from build123d import *

# Parameters (mm, degrees)
F1_DEPTH = 20
F2_W     = 20
F2_H     = 20
F3_DEPTH = 20
F5_D     = 13.2
F7_DEPTH = 20


with BuildPart() as f1:
    # F0 (on Front) → F1 (new body)
    with BuildSketch(Plane.XZ):
        Polygon((-4.964183461, 2), (-4.964183461, 0), (2.535816539, 0), (2.535816539, 2), (6.453912527, 2), (6.453912527, 4), (2.535816539, 8), (-4.964183461, 8), (-8.8822794489, 4), (-8.8822794489, 2), align=None)
        Polygon((2.535816539, 0), (-4.964183461, 0), (-8.8822794489, 0), (-8.8822794489, -55), (6.453912527, -55), (6.453912527, 0), align=None)
    extrude(amount=F1_DEPTH)

    # F2 (on face) → F3 (join)
    with BuildSketch(Plane.YZ.offset(6.453912527)):
        with Locations((-10, -45)):
            Rectangle(F2_W, F2_H)
    extrude(amount=F3_DEPTH)

    # F5 (through all)
    with Locations(Plane.YZ.offset(26.453912527)):
        with Locations((-10, -45)):
            Hole(F5_D / 2)

    # F6 (on face) → F7 (join)
    with BuildSketch(Plane.XZ.offset(20)):
        Polygon((6.453912527, -35), (26.453912527, -35), (6.453912527, 0), align=None)
    extrude(amount=-F7_DEPTH)


solid = f1.part
Could you check a few things on this model? Use its own coordinates, in mm. A direction names the side the tool comes from. Give positions to 0.01 mm unless a question says otherwise; leave off trailing zeros. Order: outer loops, then holes, each group sorted by start corner. A loop starts at its lowest first (then second) coordinate and runs counter-clockwise, first axis right, second up.
Item 1: If we section it at B-B, the plane x = 5: Write out the boundary of the cut face in (y, z).
Item 2: For faces 1 (the face through (9, -10, -55)), 2 (the face through (-4.964, -10, 1)), 3 (the face through (6.454, -10, 3)), 4 (the face through (4, -10, 2)), 5 (the face through (-8.882, -10, 3)), which set-ups out of +Z, -Z, +X, -X, +Y, -Y let a thin tool reach every point of the face, with its end or its side?
Item 3: If we section it at C-C, the plane z = -45: Write out the boundary of the cut face in (x, y), plus the area to 3 significant figures.
Item 4: I'm going to push flat-ended pins straight in: pin 1 (8 mm diameter, centred on y = -10, z = -45, fed in from +X); pin 2 (1 mm diameter, centred on y = -10.5, z = 1, fed in from -X); pin 3 (2 mm diameter, centred on x = -6.5, y = -9, fed in from +Z); pin 4 (2 mm diameter, centred on x = 4.5, y = -12, fed in from +Z). Where does each tip first touch, or does it pass through?
Item 5: I need wall thicknesses on line 1 (Z direction, x = -1, y = -10); line 2 (Z direction, x = 3.5, y = -12.5); line 3 (Z direction, x = 5, y = -10). Which ranges of each line are inside material? Lowest first, please.
Item 6: If we section it at A-A, the plane y = -10: Write out the boundary of the cut face in (x, z).
Item 7: If we mould it in two halves opening along Z, with no side actions, what happens to faces 6 (the face through (5, -10, 0)), 7 (the face through (-6.896, -9.86, 6.028)), 8 (the face through (26.454, -17, -45)), 9 (the face through (8.538, -4.762, -49.016))? For each: pulls with the +Z half, pulls with the -Z half, needs draft (parallel to the pull), parting line crosses it, or undercut.
Item 8: If we section it at D-D, the plane x = 24: Write out the boundary of the cut face in (y, z), plus the area to 3 significant figures.
Values:
1. outline: (-20, -55) - (0, -55) - (0, 0) - (-20, 0) - close; (-20, 2) - (0, 2) - (0, 5.48) - (-20, 5.48) - close; hole circle Ø13.2 at (-10, -45)
2. face 1: -Z, +X, -X, +Y, -Y
2. face 2: -X, +Y, -Y
2. face 3: +Z, +X, +Y, -Y
2. face 4: +X, +Y, -Y
2. face 5: +Z, -Z, -X, +Y, -Y
3. outline: (-8.88, -20) - (26.45, -20) - (26.45, -16.6) - (-8.88, -16.6) - close; (-8.88, -3.4) - (26.45, -3.4) - (26.45, 0) - (-8.88, 0) - close
3. area: 240 mm2
4. pin 1: passes through
4. pin 2: stops at x = -4.96
4. pin 3: stops at z = 7.45
4. pin 4: stops at z = 7.02
5. line 1: z = -55 to -51.6, -38.4 to 8
5. line 2: z = -55 to -51.11, -38.89 to 0, 2 to 7.02
5. line 3: z = -55 to -51.6, -38.4 to 0, 2 to 5.48
6. outline: (-8.88, -55) - (26.45, -55) - (26.45, -51.6) - (-8.88, -51.6) - close; (-8.88, -38.4) - (26.45, -38.4) - (26.45, -35) - (6.45, 0) - (2.54, 0) - (2.54, 2) - (6.45, 2) - (6.45, 4) - (2.54, 8) - (-4.96, 8) - (-8.88, 4) - (-8.88, 2) - (-4.96, 2) - (-4.96, 0) - (-8.88, 0) - close
7. face 6: undercut
7. face 7: pulls with the +Z half
7. face 8: needs draft
7. face 9: undercut
8. outline: (-20, -55) - (0, -55) - (0, -30.71) - (-20, -30.71) - close; hole circle Ø13.2 at (-10, -45)
8. area: 349 mm2
